```python
from build123d import *

# Parameters (mm, degrees)
BOSS_EXTRUDE1_DEPTH = 60.869805
BOSS_EXTRUDE2_START = -5
BOSS_EXTRUDE2_DEPTH = 5
FILLET1_R           = 10
SKETCH3_R           = 4.999999999999958
SKETCH3_R_2         = 4.999999999999997
SKETCH3_R_3         = 4.999999999999978
SKETCH3_R_4         = 4.999999999999986
SKETCH3_R_5         = 4.999999999999999
SKETCH3_R_6         = 5.0000000000000036
SKETCH3_R_7         = 4.999999999999983
SKETCH3_R_8         = 4.999999999999977
SKETCH3_R_9         = 5.000000000000012
SKETCH3_R_10        = 4.999999999999975
SKETCH3_R_11        = 4.9999999999999885
SKETCH3_R_12        = 4.999999999999973
SKETCH3_R_13        = 4.999999999999992
SKETCH3_R_14        = 4.999999999999971
SKETCH3_R_15        = 4.999999999999981
SKETCH3_R_16        = 4.999999999999987
SKETCH3_R_17        = 5.000000000001771
SKETCH3_R_18        = 4.9999999999999964
SKETCH3_R_19        = 4.999999999999843
SKETCH3_R_20        = 4.999999999999972
SKETCH3_R_21        = 5.000000000000026
SKETCH3_R_22        = 5.000000000000054
SKETCH3_R_23        = 5.000000000000019
SKETCH3_R_24        = 5.000000000000072
SKETCH3_R_25        = 4.999999999999844
SKETCH3_R_26        = 4.99999999999993
SKETCH3_R_27        = 5.000000000000166
SKETCH3_R_28        = 4.999999999999691
SKETCH3_R_29        = 5.000000000000506
SKETCH3_R_30        = 4.999999999999985
SKETCH3_R_31        = 4.999999999999989
SKETCH3_R_32        = 5.00000000000002
SKETCH3_R_33        = 4.999999999999994
SKETCH3_R_34        = 5.000000000000028
SKETCH3_R_35        = 4.99999999999996
SKETCH3_R_36        = 5.000000000000008
SKETCH3_R_37        = 5.000000000000001
SKETCH3_R_38        = 5.000000000000018
SKETCH3_R_39        = 5.000000000000002
SKETCH3_R_40        = 4.99999999999998
CUT_EXTRUDE1_DEPTH  = 5


with BuildPart() as part:
    # Sketch1 → Boss-Extrude1 (new body)
    with BuildSketch(Plane(origin=(0, 0, 0), x_dir=(0, 0, -1), z_dir=(1, 0, 0))):
        with BuildLine():
            Line((-101.5, -73.52493948763251), (-101.5, 94.95731051236748))
            ThreePointArc((-101.5, 94.95731051236748), (2.875e-14, 196.45731051236748), (101.5, 94.95731051236748))
            Line((101.5, 94.95731051236748), (101.5, -73.52493948763251))
            ThreePointArc((101.5, -73.52493948763251), (-1.865e-14, -175.0249394876325), (-101.5, -73.52493948763251))
        make_face()
        with BuildLine():
            Line((-91.5, -73.52493948763251), (-91.5, 94.95731051236748))
            ThreePointArc((-91.5, 94.95731051236748), (2.592e-14, 186.45731051236748), (91.5, 94.95731051236748))
            Line((91.5, 94.95731051236748), (91.5, -73.52493948763251))
            ThreePointArc((91.5, -73.52493948763251), (-1.681e-14, -165.0249394876325), (-91.5, -73.52493948763251))
        make_face(mode=Mode.SUBTRACT)
    extrude(amount=BOSS_EXTRUDE1_DEPTH)

    # Sketch2 → Boss-Extrude2 (add)
    with BuildSketch(Plane(origin=(60.869805, 0, 0), x_dir=(0, 0, -1), z_dir=(1, 0, 0)).offset(BOSS_EXTRUDE2_START)):
        with BuildLine():
            Line((-126.5, 94.95731051236748), (-126.5, -73.52493948763251))
            ThreePointArc((-126.5, -73.52493948763251), (-2.324e-14, -200.0249394876325), (126.5, -73.52493948763254))
            Line((126.5, -73.52493948763254), (126.5, 94.95731051236748))
            ThreePointArc((126.5, 94.95731051236748), (3.583e-14, 221.45731051236748), (-126.5, 94.95731051236748))
        make_face()
        with BuildLine():
            Line((101.5, -73.52493948763251), (101.5, 94.9573105123675))
            ThreePointArc((101.5, 94.9573105123675), (6.22e-15, 196.45731051236748), (-101.5, 94.95731051236751))
            Line((-101.5, 94.95731051236751), (-101.5, -73.52493948763251))
            ThreePointArc((-101.5, -73.52493948763251), (-1.865e-14, -175.0249394876325), (101.5, -73.52493948763251))
        make_face(mode=Mode.SUBTRACT)
    extrude(amount=BOSS_EXTRUDE2_DEPTH)

    # Fillet1
    fillet1_edges = [part.edges().sort_by_distance(p)[0] for p in [
        (55.869805, 10.716185512367502, 101.5),
        (55.869805, -175.0249394876325, 6.22e-15),
        (55.869805, 10.716185512367502, -101.5),
        (55.869805, 196.45731051236746, -3.12e-14),
    ]]
    fillet(fillet1_edges, radius=FILLET1_R)

    # Sketch3 → Cut-Extrude1 (cut)
    with BuildSketch(Plane.ZY.offset(-55.869805)):
        with Locations((116.50000000000001, -73.52493948763254)):
            Circle(SKETCH3_R)
        with Locations((116.49999999999991, -54.5249394876325)):
            Circle(SKETCH3_R_2)
        with Locations((114.51636611317501, -94.931758313259)):
            Circle(SKETCH3_R_3)
        with Locations((116.49999999999986, -35.52493948763251)):
            Circle(SKETCH3_R_4)
        with Locations((108.6330147256083, -115.60959359843197)):
            Circle(SKETCH3_R_5)
        with Locations((116.4999999999998, -16.52493948763251)):
            Circle(SKETCH3_R_4)
        with Locations((99.05029631250127, -134.85428646284086)):
            Circle(SKETCH3_R_6)
        with Locations((116.49999999999973, 2.475060512367487)):
            Circle(SKETCH3_R_7)
        with Locations((86.09453885620829, -152.0104819724531)):
            Circle(SKETCH3_R_8)
        with Locations((116.49999999999966, 21.475060512367484)):
            Circle(SKETCH3_R_7)
        with Locations((70.20693513818516, -166.4939464657774)):
            Circle(SKETCH3_R_9)
        with Locations((116.4999999999996, 40.47506051236748)):
            Circle(SKETCH3_R_10)
        with Locations((51.92851844796862, -177.8114629304947)):
            Circle(SKETCH3_R_11)
        with Locations((116.49999999999955, 59.47506051236749)):
            Circle(SKETCH3_R_12)
        with Locations((31.88173834339966, -185.57762691726376)):
            Circle(SKETCH3_R_13)
        with Locations((116.49999999999947, 78.47506051236748)):
            Circle(SKETCH3_R_14)
        with Locations((10.749263877476684, -189.52797102600218)):
            Circle(SKETCH3_R_15)
        with Locations((116.5, 94.95731051236747)):
            Circle(SKETCH3_R_16)
        with Locations((-10.74926387747449, -189.52797102600255)):
            Circle(SKETCH3_R_17)
        with Locations((114.51636611317436, 116.36412933800038)):
            Circle(SKETCH3_R_18)
        with Locations((-31.88173834339559, -185.57762691726487)):
            Circle(SKETCH3_R_19)
        with Locations((108.63301472560718, 137.04196462317321)):
            Circle(SKETCH3_R_7)
        with Locations((-51.92851844796495, -177.81146293049648)):
            Circle(SKETCH3_R_20)
        with Locations((99.05029631249955, 156.28665748758178)):
            Circle(SKETCH3_R_21)
        with Locations((-70.20693513818196, -166.49394646577989)):
            Circle(SKETCH3_R_22)
        with Locations((86.09453885620606, 173.44285299719374)):
            Circle(SKETCH3_R_23)
        with Locations((-86.09453885620559, -152.01048197245612)):
            Circle(SKETCH3_R_24)
        with Locations((70.20693513818269, 187.92631749051756)):
            Circle(SKETCH3_R_25)
        with Locations((-99.05029631249904, -134.85428646284436)):
            Circle(SKETCH3_R_26)
        with Locations((51.92851844796559, 199.24383395523438)):
            Circle(SKETCH3_R_27)
        with Locations((-108.63301472560683, -115.60959359843577)):
            Circle(SKETCH3_R_14)
        with Locations((31.88173834339691, 207.0099979420027)):
            Circle(SKETCH3_R_28)
        with Locations((-114.51636611317423, -94.93175831326297)):
            Circle(SKETCH3_R_7)
        with Locations((10.749263877472986, 210.96034205074073)):
            Circle(SKETCH3_R_29)
        with Locations((-116.5, -73.52493948763251)):
            Circle(SKETCH3_R_30)
        with Locations((-10.74926387747589, 210.96034205074054)):
            Circle(SKETCH3_R_2)
        with Locations((-116.50000000000006, -54.5249394876325)):
            Circle(SKETCH3_R_31)
        with Locations((-31.881738343398844, 207.0099979420022)):
            Circle(SKETCH3_R_32)
        with Locations((-116.50000000000014, -35.52493948763251)):
            Circle(SKETCH3_R_33)
        with Locations((-51.92851844796793, 199.24383395523336)):
            Circle(SKETCH3_R_34)
        with Locations((-116.50000000000016, -16.52493948763253)):
            Circle(SKETCH3_R_35)
        with Locations((-70.20693513818448, 187.9263174905162)):
            Circle(SKETCH3_R_14)
        with Locations((-116.50000000000026, 2.4750605123674947)):
            Circle(SKETCH3_R_16)
        with Locations((-86.09453885620772, 173.44285299719198)):
            Circle(SKETCH3_R_36)
        with Locations((-116.50000000000033, 21.47506051236749)):
            Circle(SKETCH3_R_16)
        with Locations((-99.05029631250082, 156.28665748757987)):
            Circle(SKETCH3_R_37)
        with Locations((-116.50000000000041, 40.47506051236749)):
            Circle(SKETCH3_R_2)
        with Locations((-108.63301472560802, 137.04196462317103)):
            Circle(SKETCH3_R_38)
        with Locations((-116.50000000000045, 59.475060512367506)):
            Circle(SKETCH3_R_31)
        with Locations((-114.51636611317484, 116.36412933799802)):
            Circle(SKETCH3_R_39)
        with Locations((-116.50000000000051, 78.47506051236749)):
            Circle(SKETCH3_R_40)
        with Locations((-116.49999999999997, 94.9573105123675)):
            Circle(SKETCH3_R_16)
    extrude(amount=-CUT_EXTRUDE1_DEPTH, mode=Mode.SUBTRACT)


solid = part.part
```
The model under review builds one solid part; all positions refer to its coordinate system, in mm. A direction names the side the tool comes from. Round coordinates to 2 decimals unless told otherwise and drop trailing zeros. Order: outer loops, then holes, each group sorted by start corner. A loop starts at its lowest first (then second) coordinate and runs counter-clockwise, first axis right, second up. Notation, with made-up numbers: (-23.5, 55.5) -> (19.5, 55.5) arc R12 ccw to (19.5, 63.5) -> close; hole circle Ø4 at (70, -4.5). An arc over 180 degrees is marked (long way). One line per item, written item: value. Start each with the question number.
Q1. Mouldability with a two-part tool opening along Y and no side actions: class faces 3 (the face through (58.33, 76.56, 121.12)), 4 (the face through (53.02, 11.9, -104.51)) as released by +Y, released by -Y, zero draft, split by the parting line, or undercut.
Q2. Take a section at A-A (z = 0). Write out the cut boundary in (x, y), and give its area (3 significant figures).
Q3. Machinability: for faces 1 (the face through (58.335, 90.076, -117.584)), 2 (the face through (55.87, 12, -112)), which of the approach directions +Z, -Z, +X, -X, +Y, -Y give a long, thin tool a straight path to every point of the face, cutting with its end or side? Answer none if there is none.
Q4. Clearance check with flat-ended pins moving along their axes: pin 1 Ø11.5 at (y, z) = (156.29, 99.05) entering from -X; pin 2 Ø18.5 at (x, y) = (26, 20) entering from -Z; pin 3 Ø1 at (x, y) = (45.5, -148) entering from -Z. State where each tip first meets the part, or that it passes through.
Q5. Wall thickness on line 1 (Z direction, x = 27.5, y = 25); line 2 (Y direction, x = 57.5, z = 3); line 3 (Y direction, x = 36.5, z = -20): over which ranges is each line inside the solid? List them lowest first.
Q6. Take a section at B-B (x = 12). Write out the cut boundary in (y, z), and give its area (3 significant figures).
Reported:
1. face 3: undercut
1. face 4: zero draft
2. outline: (0, -175.02) -> (45.87, -175.02) arc R10 cw to (55.87, -185.02) -> (55.87, -200.02) -> (60.87, -200.02) -> (60.87, -165.02) -> (0, -165.02) -> close; (0, 186.46) -> (60.87, 186.46) -> (60.87, 221.46) -> (55.87, 221.46) -> (55.87, 206.46) arc R10 cw to (45.87, 196.46) -> (0, 196.46) -> close
2. area: 1,510 mm2
3. face 1: +X, -X
3. face 2: -X
4. pin 1: stops at x = 55.84
4. pin 2: stops at z = -101.5
4. pin 3: stops at z = -69.5
5. line 1: z = -101.5 to -91.5, 91.5 to 101.5
5. line 2: y = -199.99 to -164.98, 186.41 to 221.42
5. line 3: y = -173.03 to -162.81, 184.24 to 194.47
6. outline: (-73.52, -101.5) -> (94.96, -101.5) arc R101.5 ccw to (94.96, 101.5) -> (-73.52, 101.5) arc R101.5 ccw to start; hole (-73.52, -91.5) -> (94.96, -91.5) arc R91.5 ccw to (94.96, 91.5) -> (-73.52, 91.5) arc R91.5 ccw to start
6. area: 9,430 mm2
